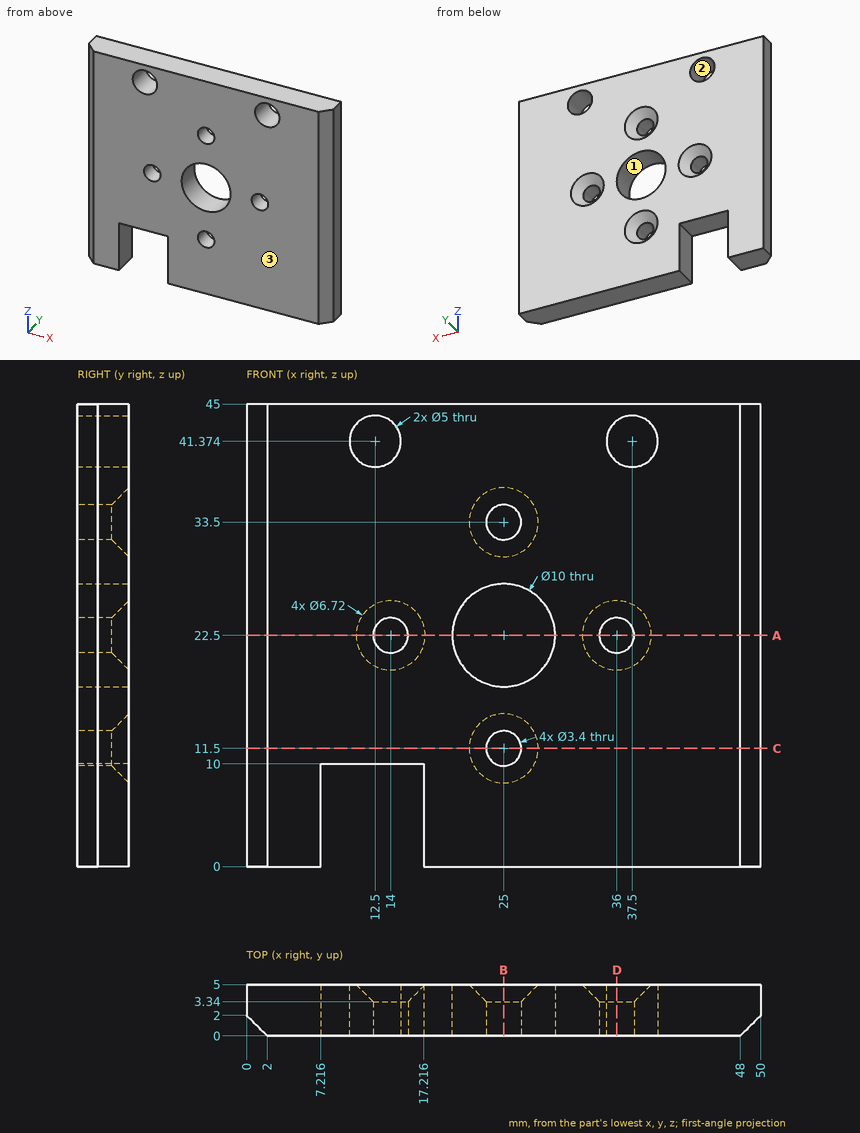
Print and shaded views of the part. All mm, measured from the part's lowest x, y and z. Coordinates: 2 decimals unless noted, no trailing zeros. Loops run counter-clockwise (first coordinate to the right, second up) from the corner with the lowest first, then second, coordinate; pieces in that order, holes last. Notation, with made-up numbers: (76.5, -19.5) - (80.5, -19.5) arc R18 cw to (80.5, -10.5) - close; hole circle Ø3 at (30, 54.25). An arc over 180 degrees is marked (long way). Use one line per item in the form item = value. Start each with the question number.
1) Band-saw the part on A-A (z = 22.5). Give the cut face in (x, y).
2) Band-saw the part on D-D (x = 36). Give the cut face in (y, z).
3) Flat gauge pins, fed straight in: pin 1 (2.5 mm diameter, centred on x = 14, z = 22.5, fed in from -Y); pin 2 (2.5 mm diameter, centred on y = 2, z = 3.5, fed in from -X); pin 3 (1 mm diameter, centred on x = 35, z = 20.5, fed in from +Y). Where does each tip first touch, or does it go through?
4) Two-plate mould, pull along Z, no slides. Class the marked faces 1, 2 and 3: +Z half, -Z half, draft (parallel to the pull), parting line (faces both ways), or undercut.
5) Band-saw the part on B-B (x = 25). Give the cut face in (y, z), and give its area (4 significant figures).
6) Drill centre lines: L1, parallel to Z at x = 25, y = 1.5; L2, parallel to Z at x = 37, y = 3.25 (1 decimal); L3, parallel to Z at x = 14, y = 2.6 (1 decimal). Where is each one in solid material? Low to high. Write a range as from..to.
7) Band-saw the part on C-C (z = 11.5). Give the cut face in (x, y).
Check values:
q1.outline = (0, 2) - (2, 0) - (12.3, 0) - (12.3, 3.34) - (10.64, 5) - (0, 5) - close; (15.7, 0) - (20, 0) - (20, 5) - (17.36, 5) - (15.7, 3.34) - close; (30, 0) - (34.3, 0) - (34.3, 3.34) - (32.64, 5) - (30, 5) - close; (37.7, 0) - (48, 0) - (50, 2) - (50, 5) - (39.36, 5) - (37.7, 3.34) - close
q2.outline = (0, 0) - (5, 0) - (5, 19.14) - (3.34, 20.8) - (0, 20.8) - close; (0, 24.2) - (3.34, 24.2) - (5, 25.86) - (5, 39.37) - (0, 39.37) - close; (0, 43.37) - (5, 43.37) - (5, 45) - (0, 45) - close
q3.pin_1 = through
q3.pin_2 = 0
q3.pin_3 = 4.38
q4.face_1 = undercut
q4.face_2 = undercut
q4.face_3 = draft
q5.outline = (0, 0) - (5, 0) - (5, 8.14) - (3.34, 9.8) - (0, 9.8) - close; (0, 13.2) - (3.34, 13.2) - (5, 14.86) - (5, 17.5) - (0, 17.5) - close; (0, 27.5) - (5, 27.5) - (5, 30.14) - (3.34, 31.8) - (0, 31.8) - close; (0, 35.2) - (3.34, 35.2) - (5, 36.86) - (5, 45) - (0, 45) - close
q5.area = 135.5 mm2
q6.L1 = 0..9.8, 13.2..17.5, 27.5..31.8, 35.2..45
q6.L2 = 0..21.1, 23.9..38.9, 43.8..45
q6.L3 = 10..20.8, 24.2..39.4, 43.4..45
q7.outline = (0, 2) - (2, 0) - (23.3, 0) - (23.3, 3.34) - (21.64, 5) - (0, 5) - close; (26.7, 0) - (48, 0) - (50, 2) - (50, 5) - (28.36, 5) - (26.7, 3.34) - close
